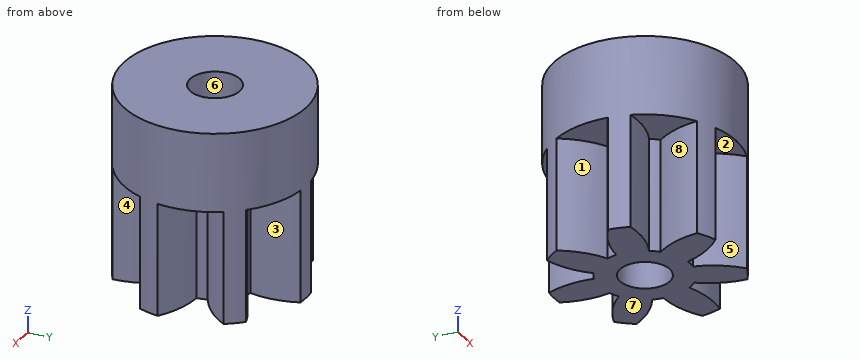
Autodesk Inventor part; units mm, degrees
ref_plane "Work Plane2" through (0, 0, 2.5) normal (0, 0, 1) x (1, 0, 0)
ref_plane "Work Plane8" through (0, 0, 0) normal (0.9009689, 0.4338837, 0) x (0, 0, 1)
ref_plane "Work Plane9" through (0, 0, 0) normal (1, 0, 0) x (0, 1, 0)
sketch "Sketch1" plane through (0, 0, 0) normal (0, 0, 1) x (1, 0, 0)
  circle A0 centre (0, 0) radius 4.0403
  dimension "d0" = 8.0806
extrude "Extrusion1" add sketch "Sketch1" along normal blind 5
ref_plane "Work Plane2" through (0, 0, 2.5) normal (0, 0, 1) x (1, 0, 0)
sketch "Sketch2" plane through (0, 0, 0) normal (0, 0, -1) x (-1, 0, 0)
  circle A0 centre (0, 0) radius 4.0403
  circle A1 centre (0, 0) radius 3.15
  dimension "d3" = 6.3
surface extrude "ピッチ円直径" sketch "Sketch2" against normal through all shown no curves A1
ref_plane "Work Plane8" through (0, 0, 0) normal (0.9009689, 0.4338837, 0) x (0, 0, 1)
ref_plane "Work Plane9" through (0, 0, 0) normal (1, 0, 0) x (0, 1, 0)
spur gear teeth "平歯車" teeth 7 pitch diameter 6.3 tip diameter 8.0806 root diameter 4.05 face width 5 start plane through (0, 0, 0) normal (0, 0, -1) x (-1, 0, 0)
sketch "スケッチ3" plane through (0, 0, 5) normal (0, 0, 1) x (1, 0, 0)
  arc A0 (-0.6688, 1.9114) -> (-1.0774, 1.7146) centre (0, 0) ccw construction
  circle A1 centre (0, 0) radius 2.025
  circle A2 centre (0, 0) radius 1.1
  circle A3 centre (0, 0) radius 4.0403
  arc A4 (1.3344, -3.8136) -> (2.1496, -3.421) centre (0, 0) ccw construction
  dimension "d49" = 2.2
extrude "押し出し2" add sketch "スケッチ3" along normal blind 3.5 contours A1 | A2
extrude "押し出し3" cut sketch "スケッチ3" along normal blind 10 from surface at -5 contours A2
extrude "押し出し4" add sketch "スケッチ3" along normal up to surface (3.5 mm away) contours A3
equation "\"d0\" = da_da"
equation "\"d1\" = da_b"
equation "\"d3\" = da_d"
equation "\"d16\" = da_aw"
equation "\"d43\" = da_aw"
equation "\"d46\" = da_aw"
properties part number "平歯車1" material "Steel"
Design review of the part built by this model. Coordinates are the model's own, in mm. Face numbers are marked on the shaded views. A direction names the side the tool comes from. Round coordinates to 2 decimals unless told otherwise and drop trailing zeros. Write each loop counter-clockwise with the first axis right and the second up, starting at its lowest first coordinate (ties: lowest second). Pieces come first, ordered by that corner, then holes.
Item 1: We need section A-A on x = 0. Write out the cut boundary in (y, z) (3 decimals).
Item 2: For probe 1 along Z at (x, y) = (-2.5, 1); probe 2 along Y at (x, z) = (-1, 4.25); probe 3 along Y at (x, z) = (3, 1), list the stretches that pass through material, from the lowest coordinate up.
Item 3: We need section D-D on y = 1.5. Write out the cut boundary in (x, z).
Item 4: For the marked faces 1, 2, 3 and 4, list the 3-axis set-ups (+Z, -Z, +X, -X, +Y, -Y) from which the entire face can be reached by the end or side of a thin tool; tool diameter is ignored.
Item 5: Clearance check with flat-ended pins moving along their axes: pin 1 Ø1.2 at (x, y) = (3, -3) entering from -Z; pin 2 Ø2 at (y, z) = (-1, 3) entering from +X. State where each tip first meets the part, or that it passes through.
Item 6: We need section C-C on y = 0. Write out the cut boundary in (x, z), and give its area (3 significant figures).
Item 7: The part is to be moulded in two halves that separate along Y. For the marked faces 5, 6, 7 and 8, say which applies: +Y half, -Y half, draft (parallel to the pull), parting line (faces both ways), or undercut.
Returned:
1. outline: (-4.04, 5) - (-2.025, 5) - (-2.025, 0) - (-1.1, 0) - (-1.1, 8.5) - (-4.04, 8.5) - close; (1.1, 0) - (4.04, 0) - (4.04, 8.5) - (1.1, 8.5) - close
2. probe 1: z = 5 to 8.5
2. probe 2: y = -3.47 to -0.46, 0.46 to 1.76
2. probe 3: y = -1.38 to 0.05, 1.55 to 2.71
3. outline: (-3.75, 5) - (-2.96, 5) - (-2.96, 0) - (2.96, 0) - (2.96, 5) - (3.75, 5) - (3.75, 8.5) - (-3.75, 8.5) - close
4. face 1: -Z, -X
4. face 2: -Z, -Y
4. face 3: -Z
4. face 4: -Z, +X
5. pin 1: stops at z = 5
5. pin 2: stops at x = 4.01
6. outline: (-4.04, 5) - (-3.14, 5) - (-3.14, 0) - (-1.1, 0) - (-1.1, 8.5) - (-4.04, 8.5) - close; (1.1, 0) - (3.14, 0) - (3.14, 5) - (4.04, 5) - (4.04, 8.5) - (1.1, 8.5) - close
6. area: 41.0 mm2
7. face 5: -Y half
7. face 6: undercut
7. face 7: draft
7. face 8: undercut
